from build123d import *

# Parameters (mm, degrees)
SKETCH2_W           = 20
SKETCH2_H           = 20
BOSS_EXTRUDE1_DEPTH = 2
SKETCH3_R           = 4.25
CUT_EXTRUDE1_DEPTH  = 15.282856857
FILLET1_R           = 10


with BuildPart() as part:
    # Sketch2 → Boss-Extrude1 (new body)
    with BuildSketch(Plane.XY):
        Rectangle(SKETCH2_W, SKETCH2_H)
    extrude(amount=BOSS_EXTRUDE1_DEPTH)

    # Sketch3 → Cut-Extrude1 (cut, through all)
    with BuildSketch(Plane.XY.offset(2)):
        with Locations((-2, 0)):
            Circle(SKETCH3_R)
    extrude(amount=-CUT_EXTRUDE1_DEPTH, mode=Mode.SUBTRACT)

    # Fillet1
    fillet1_edges = [part.edges().sort_by_distance(p)[0] for p in [
        (-10, -10, 1),
        (-10, 10, 1),
    ]]
    fillet(fillet1_edges, radius=FILLET1_R - 0.0001)  # a hair under: the kernel refuses the full size


solid = part.part
For this review, take the finished solid that the model builds, in its own axes (mm). Coordinates: 2 decimals unless noted, no trailing zeros. Loops run counter-clockwise (first coordinate to the right, second up) from the corner with the lowest first, then second, coordinate; pieces in that order, holes last. Notation, with made-up numbers: (-31, 12) - (11, 12) arc R17 cw to (11, 33) - close; hole circle Ø8 at (57.25, 52). An arc over 180 degrees is marked (long way). Use a Markdown table: item, result. Add a question column.
Item 1: For line 1 (X direction, y = -2.5, z = 1.05); line 2 (Y direction, x = -4.5, z = 1.75); line 3 (X direction, y = -1, z = 0.4), list the stretches that pass through material, from the lowest coordinate up.
Item 2: We need section C-C (y = -4). Give the boundary of the cut face in (x, z), and give its area (3 significant figures).
Item 3: We need section B-B (x = 1.25). Give the boundary of the cut face in (y, z), and give its area (3 significant figures).
Item 4: We need section D-D (y = -6.25). Give the boundary of the cut face in (x, z), and give its area (3 significant figures).
Item 5: Mouldability with a two-part tool opening along X and no side actions: class faces 1 (the face through (10, 0, 1)), 2 (the face through (-7.15, -6.99, 1.01)), 3 (the face through (2.054, 1.277, 1.014)), 4 (the face through (5, -10, 1)) as pulls with the +X half, pulls with the -X half, needs draft (parallel to the pull), parting line crosses it, or undercut.
Results list:
| question | item | result |
|---|---|---|
| 1 | line 1 | x = -9.68 to -5.44, 1.44 to 10 |
| 1 | line 2 | y = -8.93 to -3.44, 3.44 to 8.93 |
| 1 | line 3 | x = -9.95 to -6.13, 2.13 to 10 |
| 2 | outline | (-9.17, 0) - (-3.44, 0) - (-3.44, 2) - (-9.17, 2) - close; (-0.56, 0) - (10, 0) - (10, 2) - (-0.56, 2) - close |
| 2 | area | 32.6 mm^2 |
| 3 | outline | (-10, 0) - (-2.74, 0) - (-2.74, 2) - (-10, 2) - close; (2.74, 0) - (10, 0) - (10, 2) - (2.74, 2) - close |
| 3 | area | 29.0 mm^2 |
| 4 | outline | (-7.81, 0) - (10, 0) - (10, 2) - (-7.81, 2) - close |
| 4 | area | 35.6 mm^2 |
| 5 | face 1 | pulls with the +X half |
| 5 | face 2 | pulls with the -X half |
| 5 | face 3 | undercut |
| 5 | face 4 | needs draft |
